Check sheet for the modelled part. Datum: model origin and axes. Units: mm. A direction names the side the tool comes from. Round coordinates to 2 decimals unless told otherwise and drop trailing zeros. Order: outer loops, then holes, each group sorted by start corner. A loop starts at its lowest first (then second) coordinate and runs counter-clockwise, first axis right, second up. Notation, with made-up numbers: (-26.75, -4) -> (5.25, -4) arc R17 ccw to (5.25, 14) -> close; hole circle Ø1 at (64, 17). An arc over 180 degrees is marked (long way). Answer in a Markdown table with one row per item. Add a question column.
1. Sectioned sample at D-D, the plane x = 0. Count the separate pieces of the cut face and the enclosed holes in it, then the cut area to 3 significant figures.
2. Material ranges on L1, parallel to X at y = 6, z = 2 (3 decimals); L2, parallel to Z at x = 17.5, y = 9 (3 decimals); L3, parallel to Y at x = -24.5, z = 16.5 (3 decimals), recorded low to high. Write a range as from..to.
3. Sectioned sample at B-B, the plane x = 14.5. Record the boundary of the cut face in (y, z) (3 decimals), then the cut area to 3 significant figures.
4. Draft check along Z on faces 6 (the flat face through (29.854, 9.392, -7.611)), 7 (the cylindrical face through (0.33, 8.672, -6.064)), 8 (the flat face through (-26.035, 9, 0)). Enter one of: +Z half, -Z half, draft (parallel to the pull), parting line (faces both ways), or undercut.
5. Sectioned sample at A-A, the plane y = 10.16. Record the boundary of the cut face in (x, z) (3 decimals).
6. Access from +Z, -Z, +X, -X, +Y, -Y to the whole of each face (thin tool, end or side, straight path). Record for faces 1 (the cylindrical face through (0.067, 32.439, 15.622)), 2 (the flat face through (0, 14, 8.255)), 3 (the flat face through (0, 27, 8.255)), 4 (the flat face through (0, 7, -3.81)), 5 (the cylindrical face through (0.409, 30.595, -3.547)).
7. Sectioned sample at C-C, the plane y = 4.5. Record the boundary of the cut face in (x, z) (3 decimals).
8. Depth check by flat-ended pin: P1, Ø3, axis at x = 12.5, y = 8.5, coming from the +Z side (3 decimals); P2, Ø5, axis at x = 0, z = 17.145, coming from the -Y side; P3, Ø3, axis at x = 11.5, z = -4.5, coming from the +Y side. Enter the tip coordinate at first touch or a pass-through.
```python
from build123d import *
from OCP.BRepFilletAPI import BRepFilletAPI_MakeChamfer

# Parameters (mm, degrees)
SKETCH1_W           = 60.96
SKETCH1_H           = 16.51
SKETCH1_W_2         = 50.8
SKETCH1_H_2         = 6.35
BOSS_EXTRUDE1_DEPTH = 19.05
BOSS_EXTRUDE2_DEPTH = 60.96
SKETCH6_W           = 50.8
SKETCH6_H           = 6.35
CUT_EXTRUDE1_DEPTH  = 19.05
SKETCH7_R           = 1.524
CUT_EXTRUDE2_DEPTH  = 59.805251466
SKETCH8_R           = 1.524
CUT_EXTRUDE3_DEPTH  = 55.213531752
CHAMFER1_SIZE       = 2.1082
CHAMFER1_SIZE2      = 1.832630301
SKETCH9_W           = 52.07
SKETCH9_H           = 7.62
CUT_EXTRUDE4_DEPTH  = 19.05
SKETCH10_W          = 52.07
SKETCH10_H          = 7.62
CUT_EXTRUDE5_DEPTH  = 19.05
CHAMFER2_SIZE       = 1.27


with BuildPart() as part:
    # Sketch1 → Boss-Extrude1 (new body)
    with BuildSketch(Plane(origin=(0, 0, 0), x_dir=(1, 0, 0), z_dir=(0, 1, 0))):
        Rectangle(SKETCH1_W, SKETCH1_H)
        Rectangle(SKETCH1_W_2, SKETCH1_H_2, mode=Mode.SUBTRACT)
    extrude(amount=BOSS_EXTRUDE1_DEPTH)

    # Sketch5 → Boss-Extrude2 (add)
    with BuildSketch(Plane(origin=(30.48, 0, 0), x_dir=(0, 0, -1), z_dir=(1, 0, 0))):
        with BuildLine():
            Line((-8.255, 35.56), (-27.305, 35.56))
            Line((-27.305, 35.56), (-27.305, 19.05))
            Line((-27.305, 19.05), (-8.255, 19.05))
            Line((-8.255, 19.05), (8.255, 19.05))
            ThreePointArc((8.255, 19.05), (3.419332957, 30.724332957), (-8.255, 35.56))
        make_face()
    extrude(amount=-BOSS_EXTRUDE2_DEPTH)

    # Sketch6 → Cut-Extrude1 (cut)
    with BuildSketch(Plane.XY.offset(27.305)):
        with Locations((0, 27.305)):
            Rectangle(SKETCH6_W, SKETCH6_H)
    extrude(amount=-CUT_EXTRUDE1_DEPTH, mode=Mode.SUBTRACT)

    # Sketch7 → Cut-Extrude2 (cut, through all)
    with BuildSketch(Plane(origin=(0, 0, -8.255), x_dir=(-1, 0, 0), z_dir=(0, 0, -1))):
        with Locations((0, 10.16)):
            Circle(SKETCH7_R)
    extrude(amount=-CUT_EXTRUDE2_DEPTH, mode=Mode.SUBTRACT)

    # Sketch8 → Cut-Extrude3 (cut, through all)
    with BuildSketch(Plane(origin=(0, 35.56, 0), x_dir=(1, 0, 0), z_dir=(0, 1, 0))):
        with Locations(Location((0, -17.145, 0), (0, 0, 270))):
            Circle(SKETCH8_R)
    extrude(amount=-CUT_EXTRUDE3_DEPTH, mode=Mode.SUBTRACT)

    # Chamfer1: one chamfer whose edges measure the first distance from different faces: ONE call of the kernel's chamfer builder (chamfer() names one face for all edges)
    chamfer1_edges_1 = [part.edges().sort_by_distance(p)[0] for p in [
        (1.524, 10.16, 8.255),
    ]]
    chamfer1_side_1 = [part.faces().sort_by_distance(p)[0] for p in [
        (1.524, 10.16, 5.715),
    ]]
    chamfer1_edges_2 = [part.edges().sort_by_distance(p)[0] for p in [
        (0, 35.56, 15.621),
    ]]
    chamfer1_side_2 = [part.faces().sort_by_distance(p)[0] for p in [
        (0, 35.56, 8.893672381),
    ]]
    chamfer1 = BRepFilletAPI_MakeChamfer(part.part.solid().wrapped)
    for e in chamfer1_edges_1:
        chamfer1.Add(CHAMFER1_SIZE, CHAMFER1_SIZE2, e.wrapped, chamfer1_side_1[0].wrapped)  # the first distance lies on this face
    for e in chamfer1_edges_2:
        chamfer1.Add(CHAMFER1_SIZE, CHAMFER1_SIZE2, e.wrapped, chamfer1_side_2[0].wrapped)  # the first distance lies on this face
    add(Compound.cast(chamfer1.Shape()), mode=Mode.REPLACE)

    # Sketch9 → Cut-Extrude4 (cut)
    with BuildSketch(Plane.XY.offset(27.305)):
        with Locations((0, 27.305)):
            Rectangle(SKETCH9_W, SKETCH9_H)
    extrude(amount=-CUT_EXTRUDE4_DEPTH, mode=Mode.SUBTRACT)

    # Sketch10 → Cut-Extrude5 (cut)
    with BuildSketch(Plane.XZ):
        Rectangle(SKETCH10_W, SKETCH10_H)
    extrude(amount=-CUT_EXTRUDE5_DEPTH, mode=Mode.SUBTRACT)

    # Chamfer2
    chamfer2_edges = [part.edges().sort_by_distance(p)[0] for p in [
        (30.48, 30.724332957, -3.419332957),
        (30.48, 35.56, 17.78),
        (-30.48, 30.724332957, -3.419332957),
        (-30.48, 35.56, 17.78),
        (-30.48, 9.525, -8.255),
        (30.48, 9.525, -8.255),
    ]]
    chamfer(chamfer2_edges, length=CHAMFER2_SIZE)


solid = part.part
```
Answer key:
| question | item | result |
|---|---|---|
| 1 | separate pieces | 5 |
| 1 | enclosed holes | 0 |
| 1 | area | 491 mm² |
| 2 | L1 | x = -30.48..-26.035, 26.035..30.48 |
| 2 | L2 | z = -8.255..-3.81, 3.81..8.255 |
| 2 | L3 | y = 19.05..23.495, 31.115..35.56 |
| 3 | outline | (0, -8.255) -> (19.05, -8.255) arc R16.51 ccw to (35.56, 8.255) -> (35.56, 27.305) -> (31.115, 27.305) -> (31.115, 8.255) -> (23.495, 8.255) -> (23.495, 27.305) -> (19.05, 27.305) -> (19.05, 8.255) -> (0, 8.255) -> (0, 3.81) -> (19.05, 3.81) -> (19.05, -3.81) -> (0, -3.81) -> close |
| 3 | area | 553 mm² |
| 4 | face 6 | -Z half |
| 4 | face 7 | draft |
| 4 | face 8 | undercut |
| 5 | outline | (-30.48, -6.985) -> (-29.21, -8.255) -> (-1.524, -8.255) -> (-1.524, -3.81) -> (-26.035, -3.81) -> (-26.035, 3.81) -> (-1.524, 3.81) -> (-1.524, 6.147) -> (-3.357, 8.255) -> (-30.48, 8.255) -> close; (1.524, -8.255) -> (29.21, -8.255) -> (30.48, -6.985) -> (30.48, 8.255) -> (3.357, 8.255) -> (1.524, 6.147) -> (1.524, 3.81) -> (26.035, 3.81) -> (26.035, -3.81) -> (1.524, -3.81) -> close |
| 6 | face 1 | +Y, -Y |
| 6 | face 2 | +Z, +X, -X, -Y |
| 6 | face 3 | +Z |
| 6 | face 4 | -Y |
| 6 | face 5 | -Z, +X, -X, +Y |
| 7 | outline | (-30.48, -6.985) -> (-29.21, -8.255) -> (29.21, -8.255) -> (30.48, -6.985) -> (30.48, 8.255) -> (-30.48, 8.255) -> close; hole (-26.035, -3.81) -> (26.035, -3.81) -> (26.035, 3.81) -> (-26.035, 3.81) -> close |
| 8 | P1 | stops at z = 8.255 |
| 8 | P2 | stops at y = 19.05 |
| 8 | P3 | stops at y = 31.13 |
